from build123d import *

# Parameters (mm, degrees)
F1_DEPTH = 25.4


with BuildPart() as f1:
    # F0 (on Front) → F1 (new body)
    with BuildSketch(Plane.XZ):
        with BuildLine():
            Line((38.1, 19.05), (38.1, 76.2))
            Line((38.1, 76.2), (-38.1, 76.2))
            Line((-38.1, 76.2), (-38.1, 19.05))
            ThreePointArc((-38.1, 19.05), (-24.6296158184, 13.4703841816), (-19.05, 0))
            ThreePointArc((-19.05, 0), (-24.6296158184, -13.4703841816), (-38.1, -19.05))
            Line((-38.1, -19.05), (-38.1, -76.2))
            Line((-38.1, -76.2), (38.1, -76.2))
            Line((38.1, -76.2), (38.1, -19.05))
            ThreePointArc((38.1, -19.05), (19.05, 0), (38.1, 19.05))
        make_face()
        with BuildLine():
            ThreePointArc((57.15, 0), (51.5703841816, 13.4703841816), (38.1, 19.05))
            Line((38.1, 19.05), (38.1, -19.05))
            ThreePointArc((38.1, -19.05), (51.5703841816, -13.4703841816), (57.15, 0))
        make_face()
        with BuildLine():
            Line((38.1, -19.05), (38.1, 19.05))
            ThreePointArc((38.1, 19.05), (19.05, 0), (38.1, -19.05))
        make_face()
        with BuildLine():
            ThreePointArc((-19.05, 0), (-24.6296158184, 13.4703841816), (-38.1, 19.05))
            Line((-38.1, 19.05), (-38.1, -19.05))
            ThreePointArc((-38.1, -19.05), (-24.6296158184, -13.4703841816), (-19.05, 0))
        make_face()
        with BuildLine():
            Line((-38.1, -19.05), (-38.1, 19.05))
            ThreePointArc((-38.1, 19.05), (-57.15, 0), (-38.1, -19.05))
        make_face()
    extrude(amount=-F1_DEPTH)


solid = f1.part
CAD build for the part. Positions are in the model's coordinates, mm. A direction names the side the tool comes from. Round coordinates to 2 decimals unless told otherwise and drop trailing zeros. Write each loop counter-clockwise with the first axis right and the second up, starting at its lowest first coordinate (ties: lowest second). Pieces come first, ordered by that corner, then holes.
(1) Slice it at C-C, the plane x = 40. Write the cut outline in (y, z), and give its area (3 significant figures).
(2) Slice it at B-B, the plane z = 29.5. Write the cut outline in (x, y).
(3) Slice it at A-A, the plane y = 10.5. Write the cut outline in (x, z).
(4) Probe line 1 along X through (y, z) = (14.5, -52); line 2 along X through (y, z) = (23.75, -10.5). List the from-to ranges inside material, lowest first.
(5) 3-axis set-ups, long thin cutter, end or side, ignore diameter. For faces 1 (the face through (-38.1, 13, 48)), 2 (the face through (38.1, 13, 47)), 3 (the face through (-38.1, 13, -47)), 4 (the face through (38.1, 13, -48)), 5 (the face through (-1, 0, 1)): which of +Z, -Z, +X, -X, +Y, -Y reach the whole face in a straight line?
(6) Drop flat-ended pins along their axis: P1, Ø12.5, axis at y = 16, z = 51, coming from the -X side; P2, Ø2, axis at y = 13, z = -32, coming from the +X side; P3, Ø3, axis at y = 4, z = 4.5, coming from the -X side; P4, Ø2, axis at x = -12.5, z = 61, coming from the -Y side. Give the stop position or say it passes through.
From the geometry:
1. outline: (0, -18.96) - (25.4, -18.96) - (25.4, 18.96) - (0, 18.96) - close
1. area: 963 mm2
2. outline: (-38.1, 0) - (38.1, 0) - (38.1, 25.4) - (-38.1, 25.4) - close
3. outline: (-38.1, -76.2) - (38.1, -76.2) - (38.1, -19.05) arc R19.05 ccw to (38.1, 19.05) - (38.1, 76.2) - (-38.1, 76.2) - (-38.1, 19.05) arc R19.05 ccw to (-38.1, -19.05) - close
4. line 1: x = -38.1 to 38.1
4. line 2: x = -54 to 54
5. face 1: +Z, -X, +Y, -Y
5. face 2: +Z, +X, +Y, -Y
5. face 3: -Z, -X, +Y, -Y
5. face 4: -Z, +X, +Y, -Y
5. face 5: +Z, -Z, +X, -X, -Y
6. P1: stops at x = -38.1
6. P2: stops at x = 38.1
6. P3: stops at x = -56.91
6. P4: stops at y = 0
